Verification items for the finished model (mm, model axes). A direction names the side the tool comes from. Coordinates: 2 decimals unless noted, no trailing zeros. Write each loop counter-clockwise with the first axis right and the second up, starting at its lowest first coordinate (ties: lowest second). Pieces come first, ordered by that corner, then holes. Notation, with made-up numbers: (23, 8) -> (41, 8) arc R21 ccw to (41, 18) -> close; hole circle Ø8 at (-32, -22.5). An arc over 180 degrees is marked (long way). Answer in a Markdown table with one row per item.
```python
from build123d import *

# Parameters (mm, degrees)
SKETCH1_W               = 74
SKETCH1_H               = 40
BOSS_EXTRUDE1_DEPTH     = 32
SKETCH2_W               = 70
SKETCH2_H               = 36
CUT_EXTRUDE1_DEPTH      = 21
SKETCH3_W               = 44
SKETCH3_H               = 32
CUT_EXTRUDE2_DEPTH      = 6
CUT_EXTRUDE3_DEPTH      = 35
CUT_EXTRUDE3_DEPTH_BACK = 20
SKETCH4_R               = 6.375
SKETCH5_W               = 5
SKETCH5_H               = 5
BOSS_EXTRUDE2_DEPTH     = 5
SKETCH6_W               = 8
SKETCH6_H               = 24
CUT_EXTRUDE4_DEPTH      = 5
SKETCH7_R               = 2.85
CUT_EXTRUDE5_DEPTH      = 5
SKETCH8_W               = 9
SKETCH8_H               = 4
CUT_EXTRUDE6_DEPTH      = 5
FILLET1_R               = 2.5


with BuildPart() as part:
    # Sketch1 → Boss-Extrude1 (new body)
    with BuildSketch(Plane.XY):
        with Locations((37, 20)):
            Rectangle(SKETCH1_W, SKETCH1_H)
    extrude(amount=BOSS_EXTRUDE1_DEPTH)

    # Sketch2 → Cut-Extrude1 (cut)
    with BuildSketch(Plane.XY.offset(32)):
        with Locations((37, 20)):
            Rectangle(SKETCH2_W, SKETCH2_H)
    extrude(amount=-CUT_EXTRUDE1_DEPTH, mode=Mode.SUBTRACT)

    # Sketch3 → Cut-Extrude2 (cut)
    with BuildSketch(Plane.XY.offset(11)):
        with Locations((37, 20)):
            Rectangle(SKETCH3_W, SKETCH3_H)
    extrude(amount=-CUT_EXTRUDE2_DEPTH, mode=Mode.SUBTRACT)

    # Sketch4 → Cut-Extrude3 (cut, two sides: drawn at the far end of the back side and taken through both)
    with BuildSketch(Plane.XY.offset(5).offset(-CUT_EXTRUDE3_DEPTH_BACK)):
        with Locations(Location((13.5, 20, 0), (0, 0, 76.391039369))):
            Circle(SKETCH4_R)
        with Locations(Location((60.5, 20, 0), (0, 0, 103.608960631))):
            Circle(SKETCH4_R)
    extrude(amount=CUT_EXTRUDE3_DEPTH + CUT_EXTRUDE3_DEPTH_BACK, mode=Mode.SUBTRACT)

    # Sketch5 → Boss-Extrude2 (add)
    with BuildSketch(Plane.XY.offset(11)):
        with Locations((4.5, 35.5)):
            Rectangle(SKETCH5_W, SKETCH5_H)
        with Locations((69.5, 36.123202266)):
            Rectangle(SKETCH5_W, SKETCH5_H)
        with Locations((69.5, 4.5)):
            Rectangle(SKETCH5_W, SKETCH5_H)
        with Locations((4.5, 4.5)):
            Rectangle(SKETCH5_W, SKETCH5_H)
    extrude(amount=BOSS_EXTRUDE2_DEPTH)

    # Sketch6 → Cut-Extrude4 (cut)
    with BuildSketch(Plane(origin=(74, 0, 0), x_dir=(0, 0, -1), z_dir=(1, 0, 0))):
        with Locations((-22, 20)):
            Rectangle(SKETCH6_W, SKETCH6_H)
    extrude(amount=-CUT_EXTRUDE4_DEPTH, mode=Mode.SUBTRACT)

    # Sketch7 → Cut-Extrude5 (cut)
    with BuildSketch(Plane.ZY):
        with Locations((16, 20.079680134)):
            Circle(SKETCH7_R)
    extrude(amount=-CUT_EXTRUDE5_DEPTH, mode=Mode.SUBTRACT)

    # Sketch8 → Cut-Extrude6 (cut)
    with BuildSketch(Plane(origin=(0, 40, 0), x_dir=(1, 0, 0), z_dir=(0, 1, 0))):
        with Locations((37, -16)):
            Rectangle(SKETCH8_W, SKETCH8_H)
    extrude(amount=-CUT_EXTRUDE6_DEPTH, mode=Mode.SUBTRACT)

    # Fillet1
    fillet1_edges = [part.edges().sort_by_distance(p)[0] for p in [
        (0, 40, 16),
        (74, 40, 16),
        (74, 0, 16),
        (0, 0, 16),
    ]]
    fillet(fillet1_edges, radius=FILLET1_R)


solid = part.part
```
1. Depth check by flat-ended pin: P1, Ø20.5, axis at x = 60.5, y = 20, coming from the -Z side; P2, Ø2, axis at x = 73, z = 22.5, coming from the -Y side; P3, Ø2, axis at x = 73, z = 23, coming from the +Y side; P4, Ø6, axis at x = 9.5, y = 24.5, coming from the +Z side. Enter the tip coordinate at first touch or a pass-through.
Geometry says:
| item | result |
|---|---|
| P1 | z = 0 |
| P2 | y = 0.05 |
| P3 | y = 39.95 |
| P4 | z = 11 |
2. Mould release check, pull along X, two halves, no side actions. Record for faces 4 (the cylindrical face through (73.248, 0.713, 16.224)), 5 (the flat face through (34, 1, 32)), 6 (the cylindrical face through (66.874, 20.121, 4.201)): released by +X, released by -X, zero draft, split by the parting line, or undercut.
Geometry says:
| item | result |
|---|---|
| face 4 | released by +X |
| face 5 | zero draft |
| face 6 | undercut |
3. Section check C-C, the plane z = 27. Record the boundary of the cut face in (x, y).
Geometry says:
| item | result |
|---|---|
| outline | (0, 2.5) arc R2.5 ccw to (2.5, 0) -> (71.5, 0) arc R2.5 ccw to (74, 2.5) -> (74, 37.5) arc R2.5 ccw to (71.5, 40) -> (2.5, 40) arc R2.5 ccw to (0, 37.5) -> close; hole (2, 2) -> (72, 2) -> (72, 38) -> (2, 38) -> close |
4. Section check D-D, the plane y = 12.5. Record the boundary of the cut face in (x, z).
Geometry says:
| item | result |
|---|---|
| outline | (0, 0) -> (74, 0) -> (74, 18) -> (72, 18) -> (72, 11) -> (59, 11) -> (59, 5) -> (15, 5) -> (15, 11) -> (2, 11) -> (2, 32) -> (0, 32) -> close; (72, 26) -> (74, 26) -> (74, 32) -> (72, 32) -> close |
5. Thickness scan on line 1 (Y direction, x = 41, z = 19.5); line 2 (X direction, y = 20, z = 2.5) (3 decimals); line 3 (Y direction, x = 30, z = 9). Record the ranges inside material, lowest first. Write a range as from..to.
Geometry says:
| item | result |
|---|---|
| line 1 | 0..2, 38..40 |
| line 2 | 0..7.125, 19.875..54.125, 66.875..74 |
| line 3 | 0..4, 36..40 |
6. Section check A-A, the plane z = 2.5. Record the boundary of the cut face in (x, y) (3 decimals), plus the area to 3 significant figures.
Geometry says:
| item | result |
|---|---|
| outline | (0, 2.5) arc R2.5 ccw to (2.5, 0) -> (71.5, 0) arc R2.5 ccw to (74, 2.5) -> (74, 37.5) arc R2.5 ccw to (71.5, 40) -> (2.5, 40) arc R2.5 ccw to (0, 37.5) -> close; hole circle Ø12.75 at (13.5, 20); hole circle Ø12.75 at (60.5, 20) |
| area | 2,700 mm^2 |
7. Tool access check on faces 1 (the flat face through (73, 32, 22)), 2 (the flat face through (37, 39, 14)), 3 (the flat face through (59, 31, 8)). Record the directions out of +Z, -Z, +X, -X, +Y, -Y that give a thin tool (end or side, any length) a straight path to the whole face; none if there is none.
Geometry says:
| item | result |
|---|---|
| face 1 | +X |
| face 2 | +Y |
| face 3 | +Z |
8. Section check B-B, the plane x = 60.5. Record the boundary of the cut face in (y, z) (3 decimals), plus the area to 3 significant figures.
Geometry says:
| item | result |
|---|---|
| outline | (0, 0) -> (13.625, 0) -> (13.625, 11) -> (2, 11) -> (2, 32) -> (0, 32) -> close; (26.375, 0) -> (40, 0) -> (40, 32) -> (38, 32) -> (38, 11) -> (26.375, 11) -> close |
| area | 384 mm^2 |
